Answer from the drawing. Dimensions are ordinates in mm from the lowest x, y and z of the part. A direction names the side the tool comes from. Give positions to 0.01 mm unless a question says otherwise; leave off trailing zeros. Order: outer loops, then holes, each group sorted by start corner. A loop starts at its lowest first (then second) coordinate and runs counter-clockwise, first axis right, second up.
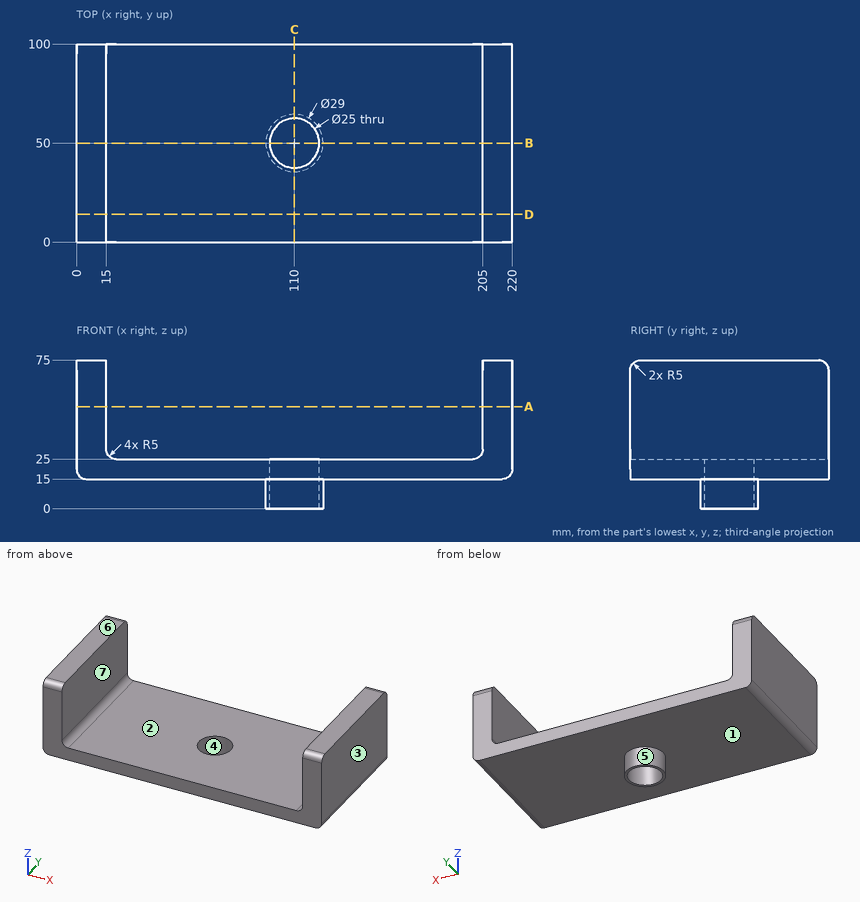
1) Given pin 1 (8 mm diameter, centred on x = 119, y = 85, fed in from -Z); pin 2 (4 mm diameter, centred on y = 36.5, z = 8, fed in from +X); pin 3 (20 mm diameter, centred on x = 110, y = 50, fed in from +Z), each flat-ended and moving along its own axis, determine where each tip first touches the part or whether it passes through.
Final values:
pin 1: stops at z = 15
pin 2: stops at x = 118.83
pin 3: passes through
2) The part is cut by section C-C on x = 110. Determine the outline of the cut face in (y, z), and give its area (3 significant figures).
Final values:
outline: (0, 15) - (35.5, 15) - (35.5, 0) - (37.5, 0) - (37.5, 25) - (0, 25) - close; (62.5, 0) - (64.5, 0) - (64.5, 15) - (100, 15) - (100, 25) - (62.5, 25) - close
area: 810 mm2
3) The part is cut by section A-A on z = 51.5. Determine the outline of the cut face in (x, y).
Final values:
outline: (0, 0) - (15, 0) - (15, 100) - (0, 100) - close; (205, 0) - (220, 0) - (220, 100) - (205, 100) - close
4) Consider L1, parallel to Y at x = 110, z = 12.25; L2, parallel to X at y = 67, z = 33; L3, parallel to Y at x = 110, z = 16. Determine where each line is inside the solid, lowest interval first.
Final values:
L1: y = 35.5 to 37.5, 62.5 to 64.5
L2: x = 0 to 15, 205 to 220
L3: y = 0 to 37.5, 62.5 to 100
5) A tool of negligible diameter and unlimited length cuts with its end or side. For the marked faces 5, 6 and 7, from which of +Z, -Z, +X, -X, +Y, -Y can it reach the whole face along a straight path? Write none if from no direction.
Final values:
face 5: -Z
face 6: +Z, +X, -X, +Y, -Y
face 7: +Z, +Y, -Y
6) The part is cut by section D-D on y = 14. Determine the outline of the cut face in (x, z), and give its area (3 significant figures).
Final values:
outline: (0, 20) arc R5 ccw to (5, 15) - (215, 15) arc R5 ccw to (220, 20) - (220, 75) - (205, 75) - (205, 30) arc R5 cw to (200, 25) - (20, 25) arc R5 cw to (15, 30) - (15, 75) - (0, 75) - close
area: 3,700 mm2
7) The part is cut by section B-B on y = 50. Determine the outline of the cut face in (x, z), and give its area (3 significant figures).
Final values:
outline: (0, 20) arc R5 ccw to (5, 15) - (95.5, 15) - (95.5, 0) - (97.5, 0) - (97.5, 25) - (20, 25) arc R5 cw to (15, 30) - (15, 75) - (0, 75) - close; (122.5, 0) - (124.5, 0) - (124.5, 15) - (215, 15) arc R5 ccw to (220, 20) - (220, 75) - (205, 75) - (205, 30) arc R5 cw to (200, 25) - (122.5, 25) - close
area: 3,510 mm2
8) For a pull along X with two mould halves and no side action, classify the marked faces 1, 2, 3 and 4 as released by +X, released by -X, zero draft, split by the parting line, or undercut.
Final values:
face 1: zero draft
face 2: undercut
face 3: released by +X
face 4: undercut
